Study the drawing (mm; zero at the part's minimum x, y, z) and answer. Round coordinates to 2 decimals unless told otherwise and drop trailing zeros. Order: outer loops, then holes, each group sorted by start corner. A loop starts at its lowest first (then second) coordinate and runs counter-clockwise, first axis right, second up. Notation, with made-up numbers: (89, -12) -> (114, -12) arc R4 cw to (114, -6) -> close; hole circle Ø4 at (46.25, 15.5). An arc over 180 degrees is marked (long way). Use one line per item in the form item = value.
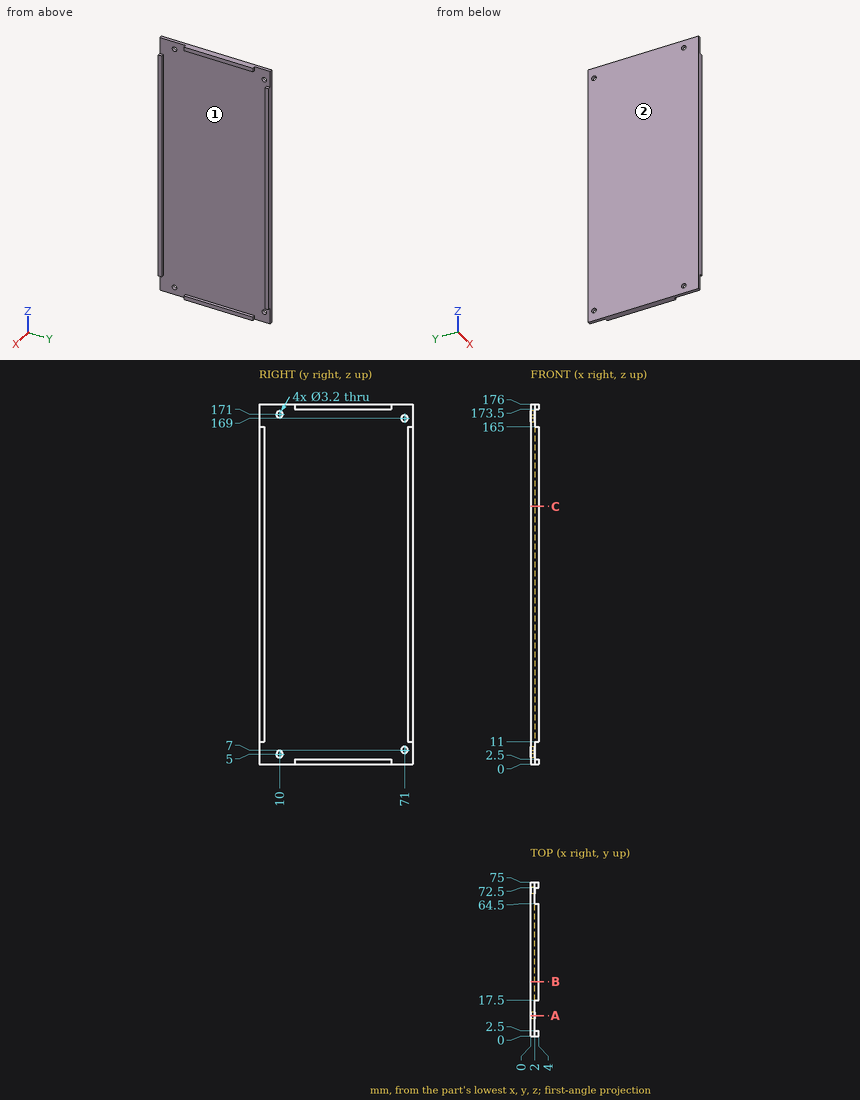
Item 1: Determine the mould class of the marked faces 1 and 2 for opening direction Z: released by +Z, released by -Z, zero draft, split by the parting line, or undercut.
Findings:
face_1 = undercut
face_2 = zero draft
Item 2: Consider line 1 along Z through (x, y) = (1.35, 71); line 2 along Y through (x, z) = (2.5, 145); line 3 along Y through (x, z) = (1.05, 169). Determine where each line is inside the solid, lowest interval first.
Findings:
line_1 = 0 to 5.4, 8.6 to 167.4, 170.6 to 176
line_2 = 0 to 2.5, 72.5 to 75
line_3 = 0 to 69.4, 72.6 to 75
Item 3: Flat-ended cylindrical pins translate along their axes: P1, Ø22.5, axis at y = 52.5, z = 54.5, coming from the +X side; P2, Ø1.6, axis at x = 3.5, z = 1, coming from the -Y side; P3, Ø3, axis at y = 10, z = 5, coming from the -X side; P4, Ø1.6, axis at x = 3.5, z = 1, coming from the +Y side. Find the tip coordinate at first contact, or state that the pin passes through.
Findings:
P1 = 2
P2 = 17.5
P3 = through
P4 = 64.5
Item 4: The part is cut by section B-B, the plane y = 26.5. Give the vertices of the cut face in (x, z).
Findings:
outline = (0, 0) -> (4, 0) -> (4, 2.5) -> (2, 2.5) -> (2, 173.5) -> (4, 173.5) -> (4, 176) -> (0, 176) -> close
Item 5: The part is cut by section C-C, the plane z = 126. Give the vertices of the cut face in (x, y).
Findings:
outline = (0, 0) -> (4, 0) -> (4, 2.5) -> (2, 2.5) -> (2, 72.5) -> (4, 72.5) -> (4, 75) -> (0, 75) -> close
Item 6: The part is cut by section A-A, the plane y = 10. Give the vertices of the cut face in (x, z).
Findings:
outline = (0, 0) -> (2, 0) -> (2, 3.4) -> (0, 3.4) -> close; (0, 6.6) -> (2, 6.6) -> (2, 169.4) -> (0, 169.4) -> close; (0, 172.6) -> (2, 172.6) -> (2, 176) -> (0, 176) -> close
